Source: CAD feature listing. Evaluate the final solid. Frame: model axes, mm. Face numbers are marked on the shaded views. A direction names the side the tool comes from. Give positions to 0.01 mm unless a question says otherwise; leave off trailing zeros. Order: outer loops, then holes, each group sorted by start corner. A loop starts at its lowest first (then second) coordinate and runs counter-clockwise, first axis right, second up.
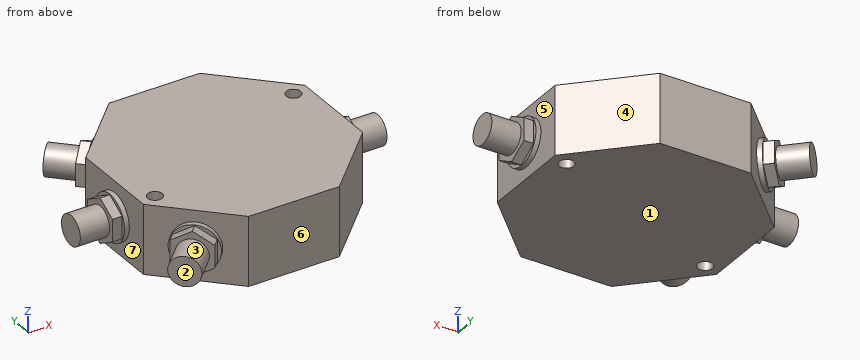
Autodesk Inventor part; units mm, degrees
ref_plane "YZ Plane" through (0, 0, 0) normal (1, 0, 0) x (0, 1, 0)
ref_plane "XZ Plane" through (0, 0, 0) normal (0, 1, 0) x (-1, 0, 0)
ref_plane "XY Plane" through (0, 0, 0) normal (0, 0, 1) x (1, 0, 0)
sketch "Sketch1" plane through (0, 0, 0) normal (0, 0, 1) x (1, 0, 0)
  line L0 (-22.55, 9.3405) -> (-9.3405, 22.55)
  line L1 (-9.3405, 22.55) -> (9.3405, 22.55)
  line L2 (9.3405, 22.55) -> (22.55, 9.3405)
  line L3 (22.55, 9.3405) -> (22.55, -9.3405)
  line L4 (22.55, -9.3405) -> (9.3405, -22.55)
  line L5 (9.3405, -22.55) -> (-9.3405, -22.55)
  line L6 (-9.3405, -22.55) -> (-22.55, -9.3405)
  line L7 (-22.55, -9.3405) -> (-22.55, 9.3405)
  point P0 (0, 0)
  point P1 (0, 0)
  point P2 (0, 22.55)
  dimension "d0" = 45.1
extrude "Extrusion1" add sketch "Sketch1" along normal blind 14.2
sketch "Sketch2" plane through (22.55, -9.3405, 0) normal (1, 0, 0) x (0, 0, -1)
  circle A0 centre (-7.1, 9.3405) radius 4.75
  line L0 (0, 0) -> (0, 18.681)
  line L1 (0, 18.681) -> (-14.2, 18.681)
  point P0 (0, 9.3405)
  point P1 (0, 9.3405)
  point P2 (-7.1, 18.681)
  dimension "d3" = 9.5
extrude "Extrusion2" add sketch "Sketch2" along normal blind 1
sketch "Sketch3" plane through (23.55, 0, 7.1) normal (1, 0, 0) x (0, 0, -1)
  line L0 (4.6188, 0) -> (2.3094, -4)
  line L1 (2.3094, -4) -> (-2.3094, -4)
  line L2 (-2.3094, -4) -> (-4.6188, 0)
  line L3 (-4.6188, 0) -> (-2.3094, 4)
  line L4 (-2.3094, 4) -> (2.3094, 4)
  line L5 (2.3094, 4) -> (4.6188, 0)
  line L6 (7.1, 9.3405) -> (-7.1, 9.3405)
  point P0 (7.1, 0)
  point P1 (0, 0)
  point P2 (0, 9.3405)
  dimension "d6" = 8
extrude "Extrusion3" add sketch "Sketch3" along normal blind 2
sketch "Sketch5" plane through (25.55, 0, 7.1) normal (1, 0, 0) x (0, 0, -1)
  circle A0 centre (0, 0) radius 3.05
  point P0 (7.1, 0)
  dimension "d9" = 6.1
extrude "Extrusion4" add sketch "Sketch5" along normal blind 6
pattern_circular "Circular Pattern1" count 2 over 135 about axis through (0, 0, -10) along (0, 0, 1) of "Extrusion2", "Extrusion3", "Extrusion4"
pattern_circular "Circular Pattern2" count 2 over 360 about axis through (0, 0, -10) along (0, 0, 1) of "Extrusion2", "Extrusion3", "Extrusion4"
pattern_circular "Circular Pattern3" count 2 over 225 about axis through (0, 0, -10) along (0, 0, 1) of "Extrusion2", "Extrusion3", "Extrusion4"
sketch "Sketch7" plane through (0, 0, 14.2) normal (0, 0, 1) x (1, 0, 0)
  circle A0 centre (19.35, 8.015) radius 1.5
  line L0 (22.55, 9.3405) -> (9.3405, 22.55)
  line L1 (22.55, 9.3405) -> (-22.55, -9.3405)
  circle A1 centre (-19.35, -8.015) radius 1.5
  point P0 (0, 0)
  dimension "d21" = 3
  dimension "d22" = 6.4
  dimension "d25" = 360
extrude "Extrusion5" cut sketch "Sketch7" against normal through all
properties part number "signal_combiner"
1) Section query B-B, the plane z = 1.5. Count the separate pieces of the cut face and the enclosed holes in it, and give its area (3 significant figures).
Report:
separate pieces: 1
enclosed holes: 2
area: 1,670 mm2
2) Section query C-C, the plane x = 6. Return the cut outline in (y, z), and give its area (3 significant figures).
Report:
outline: (-22.55, 0) - (22.55, 0) - (22.55, 14.2) - (-22.55, 14.2) - close
area: 640 mm2
3) Material intervals for L1, parallel to Y at x = -19, z = 4.5 (1 decimal); L2, parallel to X at y = 2.5, z = 1, sorted ascending.
Report:
L1: y = -21.3 to -13.4, -12.9 to -9.5, -6.6 to 12.9, 13.4 to 21.3
L2: x = -22.55 to 22.55
4) Section query A-A, the plane x = 19.35. Return the cut outline in (y, z) (1 decimal).
Report:
outline: (-12.5, 0) - (6.5, 0) - (6.5, 14.2) - (-12.5, 14.2) - close; (9.5, 0) - (12.5, 0) - (12.5, 14.2) - (9.5, 14.2) - close
5) Pin query (flat end, axial travel): pin 1 (2 mm diameter, centred on y = 12, z = 11.5, fed in from -X); pin 2 (2 mm diameter, centred on y = -19, z = 10, fed in from -X); pin 3 (6 mm diameter, centred on y = 4, z = 12.5, fed in from +X). Return the tip coordinate at first contact, or that it passes through.
Report:
pin 1: stops at x = -20.89
pin 2: stops at x = -22.73
pin 3: stops at x = 25.55
6) Draft query along X for the marked faces 1, 2, 3 and 4. Return one class per face: +X half, -X half, draft (parallel to the pull), parting line (faces both ways), or undercut.
Report:
face 1: draft
face 2: -X half
face 3: undercut
face 4: +X half
7) Reachability of the marked faces 5, 6 and 7 from +Z, -Z, +X, -X, +Y, -Y: full face, straight path, thin tool, end or side. Return the list, or none.
Report:
face 5: +X
face 6: +Z, -Z, +X, -Y
face 7: -X
